Geometry check sheet. Reference: the model listing, model coordinates, mm. A direction names the side the tool comes from. Coordinates: 2 decimals unless noted, no trailing zeros. Write each loop counter-clockwise with the first axis right and the second up, starting at its lowest first coordinate (ties: lowest second). Pieces come first, ordered by that corner, then holes. Notation, with made-up numbers: (-10, -19) -> (42, -19) arc R26 cw to (42, 7) -> close; hole circle Ø4 at (87.25, 23.25). An arc over 180 degrees is marked (long way). One line per question, with ' | ' between items.
from build123d import *

# Parameters (mm, degrees)
SKETCH_1_W                = 39.896146096
SKETCH_1_H                = 53.32653191
EXTRUDE_1_DEPTH           = 2
SKETCH_2_W                = 12
SKETCH_2_H                = 39.863647893
EXTRUDE_2_DEPTH           = 10
HOLE_WIZARD_1_D           = 4.5
HOLE_WIZARD_1_CBORE_D     = 8
HOLE_WIZARD_1_CBORE_DEPTH = 4.6
SKETCH_6_W                = 10
SKETCH_6_H                = 14
CUT_EXTRUDE_1_DEPTH       = 50.184489279
SKETCH_8_W                = 7.051926952
SKETCH_8_H                = 53.179699591
EXTRUDE_3_DEPTH           = 2
CUT_EXTRUDE_2_DEPTH       = 40.24193868
HOLE_WIZARD_2_D           = 2.4
HOLE_WIZARD_2_CBORE_D     = 4.3
HOLE_WIZARD_2_CBORE_DEPTH = 0.5
SKETCH_12_W               = 21.084425155
SKETCH_12_H               = 3
CUT_EXTRUDE_3_DEPTH       = 40.24193868
FILLET_1_R                = 3
SKETCH_13_W               = 15.522379956
SKETCH_13_H               = 43.706267889
CUT_EXTRUDE_4_DEPTH       = 40.24193868
SKETCH_14_W               = 6
SKETCH_14_H               = 11.863647893
CUT_EXTRUDE_5_DEPTH       = 4.6
SKETCH_15_W               = 6
SKETCH_15_H               = 4.5
CUT_EXTRUDE_6_DEPTH       = 50.809738004
FILLET_2_R                = 3.7
FILLET_3_R                = 3.7
SKETCH_17_W               = 11.863647893
SKETCH_17_H               = 4.6
CUT_EXTRUDE_7_DEPTH       = 4


# Some blends are built 0.0001 mm under size
with BuildPart() as part:
    # 草图1 → 凸台-拉伸1 (new body)
    with BuildSketch(Plane(origin=(0, 0, 0), x_dir=(0, 0, -1), z_dir=(1, 0, 0))):
        Rectangle(SKETCH_1_W, SKETCH_1_H)
    extrude(amount=EXTRUDE_1_DEPTH)

    # 草图2 → 凸台-拉伸2 (add)
    with BuildSketch(Plane.XZ.offset(26.663265955)):
        with Locations((6, 0.016249101)):
            Rectangle(SKETCH_2_W, SKETCH_2_H)
    extrude(amount=-EXTRUDE_2_DEPTH)

    # 打孔尺寸(%根据)内六角圆柱头螺钉的类型1 (through all)
    with Locations(Plane(origin=(6, -16.663265955, 0), x_dir=(0, 0, 1), z_dir=(0, 1, 0))):
        with Locations((0, 0)):
            CounterBoreHole(HOLE_WIZARD_1_D / 2, HOLE_WIZARD_1_CBORE_D / 2, HOLE_WIZARD_1_CBORE_DEPTH)

    # 草图6 → 切除-拉伸1 (cut, through all)
    with BuildSketch(Plane(origin=(0, -16.663265955, 0), x_dir=(1, 0, 0), z_dir=(0, 1, 0))):
        with Locations((7, 12.915574845)):
            Rectangle(SKETCH_6_W, SKETCH_6_H)
        with Locations((7, -12.948073048)):
            Rectangle(SKETCH_6_W, SKETCH_6_H)
    extrude(amount=-CUT_EXTRUDE_1_DEPTH, mode=Mode.SUBTRACT)

    # 草图8 → 凸台-拉伸3 (add)
    with BuildSketch(Plane(origin=(2, 0, 0), x_dir=(0, 0, -1), z_dir=(1, 0, 0))):
        with Locations((23.474036524, -0.073416159)):
            Rectangle(SKETCH_8_W, SKETCH_8_H)
    extrude(amount=-EXTRUDE_3_DEPTH)

    # 草图9 → 切除-拉伸2 (cut, through all)
    with BuildSketch(Plane(origin=(2, 0, 0), x_dir=(0, 0, -1), z_dir=(1, 0, 0))):
        with BuildLine():
            ThreePointArc((-10.54, 13.836734045), (-9.075533906, 17.372267951), (-5.54, 18.836734045))
            Line((-5.54, 18.836734045), (7, 18.836734045))
            ThreePointArc((7, 18.836734045), (21.142135624, 12.978869669), (27, -1.163265955))
            Line((27, -1.163265955), (27, 26.516433636))
            Line((27, 26.516433636), (19.948073048, 26.516433636))
            Line((19.948073048, 26.516433636), (19.948073048, 26.663265955))
            Line((19.948073048, 26.663265955), (-19.948073048, 26.663265955))
            Line((-19.948073048, 26.663265955), (-19.948073048, -3.722994561))
            ThreePointArc((-19.948073048, -3.722994561), (-17.113911838, 5.186324453), (-10.54, 11.834039714))
            Line((-10.54, 11.834039714), (-10.54, 13.836734045))
        make_face()
        with BuildLine():
            ThreePointArc((-5.948073048, -24.258302666), (-15.670841721, -17.590040264), (-19.948073048, -6.603537348))
            Line((-19.948073048, -6.603537348), (-19.948073048, -26.663265955))
            Line((-19.948073048, -26.663265955), (-5.948073048, -26.663265955))
            Line((-5.948073048, -26.663265955), (-5.948073048, -24.258302666))
        make_face()
    extrude(amount=-CUT_EXTRUDE_2_DEPTH, mode=Mode.SUBTRACT)

    # 打孔尺寸(%根据)内六角圆柱头螺钉的类型2 (through all)
    with Locations(Plane(origin=(2, 7.336734045, -21.650635095), x_dir=(0, 0, 1), z_dir=(1, 0, 0))):
        with Locations((0, 0), (0, 25)):
            CounterBoreHole(HOLE_WIZARD_2_D / 2, HOLE_WIZARD_2_CBORE_D / 2, HOLE_WIZARD_2_CBORE_DEPTH)

    # 草图12 → 切除-拉伸3 (cut, through all)
    with BuildSketch(Plane(origin=(2, 0, 0), x_dir=(0, 0, -1), z_dir=(1, 0, 0))):
        with Locations((16.457787423, -25.163265955)):
            Rectangle(SKETCH_12_W, SKETCH_12_H)
    extrude(amount=-CUT_EXTRUDE_3_DEPTH, mode=Mode.SUBTRACT)

    # 圆角1
    fillet_1_edges = [part.edges().sort_by_distance(p)[0] for p in [
        (1, -23.663265955, -5.915574845),
    ]]
    fillet(fillet_1_edges, radius=FILLET_1_R - 0.0001)  # a hair under: the kernel refuses the full size

    # 草图13 → 切除-拉伸4 (cut, through all)
    with BuildSketch(Plane(origin=(2, 0, 0), x_dir=(0, 0, -1), z_dir=(1, 0, 0))):
        with Locations((-13.709263026, -2.405168722)):
            Rectangle(SKETCH_13_W, SKETCH_13_H)
    extrude(amount=-CUT_EXTRUDE_4_DEPTH, mode=Mode.SUBTRACT)

    # 草图14 → 切除-拉伸5 (cut)
    with BuildSketch(Plane(origin=(0, -16.663265955, 0), x_dir=(1, 0, 0), z_dir=(0, 1, 0))):
        with Locations((9, -0.016249102)):
            Rectangle(SKETCH_14_W, SKETCH_14_H)
    extrude(amount=-CUT_EXTRUDE_5_DEPTH, mode=Mode.SUBTRACT)

    # 草图15 → 切除-拉伸6 (cut, through all)
    with BuildSketch(Plane(origin=(0, -21.263265955, 0), x_dir=(1, 0, 0), z_dir=(0, 1, 0))):
        with Locations((9, 0)):
            Rectangle(SKETCH_15_W, SKETCH_15_H)
    extrude(amount=-CUT_EXTRUDE_6_DEPTH, mode=Mode.SUBTRACT)

    # 圆角2
    # the kernel refuses this fillet: 3.7 mm, written as the material it takes off along each edge
    with BuildSketch(Plane(origin=(12, -12.013265955, -5.915574845), x_dir=(-1, 0, 0), z_dir=(0, -1, 0))) as fillet_2_piece_1:
        with BuildLine():
            CenterArc((FILLET_2_R, -FILLET_2_R), FILLET_2_R, 90, 90)
            Line((0, -FILLET_2_R), (0, 0))
            Line((0, 0), (FILLET_2_R, 0))
        make_face()
    extrude(amount=23.9, mode=Mode.SUBTRACT)
    with BuildSketch(Plane(origin=(12, -12.013265955, 5.948073048), x_dir=(-1, 0, 0), z_dir=(0, -1, 0))) as fillet_2_piece_2:
        with BuildLine():
            CenterArc((FILLET_2_R, FILLET_2_R), FILLET_2_R, 180, 90)
            Line((0, FILLET_2_R), (0, 0))
            Line((0, 0), (FILLET_2_R, 0))
        make_face()
    extrude(amount=23.9, mode=Mode.SUBTRACT)

    # 圆角3
    # the kernel refuses this fillet: 3.7 mm, written as the material it takes off along each edge
    with BuildSketch(Plane(origin=(11.25, -23.663265955, -27), x_dir=(0, 1, 0), z_dir=(-1, 0, 0))) as fillet_3_piece_1:
        with BuildLine():
            CenterArc((FILLET_3_R, -FILLET_3_R), FILLET_3_R, 90, 90)
            Line((0, -FILLET_3_R), (0, 0))
            Line((0, 0), (FILLET_3_R, 0))
        make_face()
    extrude(amount=20.5, mode=Mode.SUBTRACT)
    with BuildSketch(Plane(origin=(-9.250093996, 18.820053861, 5.948073048), x_dir=(0, -1, 0), z_dir=(1, 0, 0))) as fillet_3_piece_2:
        with BuildLine():
            CenterArc((3.683319816, 3.7), FILLET_3_R, 180, 90)
            Line((-0.016680184, 3.7), (-0.386680184, 3.7))
            ThreePointArc((-0.386680184, 3.7), (-0.386680184, 0.408073048), (-0.368765666, -0.030197406))
            Line((-0.368765666, -0.030197406), (0, -0.37))
            Line((0, -0.37), (3.683319816, -0.37))
            Line((3.683319816, -0.37), (3.683319816, 0))
        make_face()
    extrude(amount=20.500187991, mode=Mode.SUBTRACT)

    # 草图17 → 切除-拉伸7 (cut)
    with BuildSketch(Plane(origin=(6, 0, 0), x_dir=(0, 0, -1), z_dir=(1, 0, 0))):
        with Locations((-0.016249102, -18.963265955)):
            Rectangle(SKETCH_17_W, SKETCH_17_H)
    extrude(amount=-CUT_EXTRUDE_7_DEPTH, mode=Mode.SUBTRACT)


solid = part.part
1. Cross-section at A-A on x = 7.75. Record the boundary of the cut face in (y, z).
Worked answers:
outline: (-26.66, -5.92) -> (-21.26, -5.92) -> (-21.26, -2.25) -> (-26.66, -2.25) -> close; (-26.66, 2.25) -> (-21.26, 2.25) -> (-21.26, 5.95) -> (-26.66, 5.95) -> close
2. Cross-section at B-B on z = 0. Record the boundary of the cut face in (x, y).
Worked answers:
outline: (0, -26.66) -> (3.75, -26.66) -> (3.75, -21.26) -> (2, -21.26) -> (2, 18.84) -> (0, 18.84) -> close
3. Mould release check, pull along Z, two halves, no side actions. Record for faces 5 (the face through (0.986, 17.782, 4.835)), 6 (the face through (0.986, -24.519, -6.818)), 7 (the face through (0.74, 7.796, -22.759)), 8 (the face through (1, -23.663, -16)): released by +Z, released by -Z, zero draft, split by the parting line, or undercut.
Worked answers:
face 5: released by +Z | face 6: released by -Z | face 7: undercut | face 8: zero draft
4. Go/stop test with flat-tipped pins: P1, Ø10, axis at y = -10, z = -3.5, coming from the +X side; P2, Ø1.3, axis at y = -16.5, z = -22, coming from the +X side; P3, Ø2, axis at x = 1, z = -14.5, coming from the -Y side; P4, Ø1.3, axis at y = 7.5, z = -22, coming from the +X side. Record where each tip stops, or that it passes through.
Worked answers:
P1: x = 2 | P2: x = 1.5 | P3: y = -23.66 | P4: through
5. Tool access check on faces 1 (the face through (9, -24, 2.25)), 2 (the face through (7, -21.263, -3)), 3 (the face through (10.94, -23.93, 4.84)), 4 (the face through (1.75, 6.69, -19.6)). Record the directions out of +Z, -Z, +X, -X, +Y, -Y that give a thin tool (end or side, any length) a straight path to the whole face; none if there is none.
Worked answers:
face 1: +X, +Y, -Y | face 2: +Z, -Z, +X, +Y | face 3: +Z, +X, +Y, -Y | face 4: +X
6. Material ranges on line 1 (X direction, y = -4, z = -15); line 2 (Z direction, x = 5.75, y = -24); line 3 (Y direction, x = 8.5, z = -3), recorded low to high. Write a range as from..to.
Worked answers:
line 1: 0..2 | line 2: -5.92..-2.24, 2.24..5.95 | line 3: -26.66..-21.26
7. Cross-section at D-D on z = -4.5. Record the boundary of the cut face in (x, y).
Worked answers:
outline: (0, -26.66) -> (11.21, -26.66) -> (11.21, -21.26) -> (2, -21.26) -> (2, 18.84) -> (0, 18.84) -> close
8. Cross-section at C-C on y = -9. Record the boundary of the cut face in (x, z).
Worked answers:
outline: (0, -27) -> (2, -27) -> (2, 5.95) -> (0, 5.95) -> close
